Input: dimensioned drawing with shaded views. Units: mm. Origin: part minimum x, y, z. A direction names the side the tool comes from. Coordinates: 2 decimals unless noted, no trailing zeros. Loops run counter-clockwise (first coordinate to the right, second up) from the corner with the lowest first, then second, coordinate; pieces in that order, holes last.
Item 1: Ray query, line 1 along Y through (x, z) = (8, 2.75); line 2 along Y through (x, z) = (4.25, 11.25); line 3 along X through (y, z) = (13.75, 7.5). Return the intervals inside material, ascending.
Item 2: Section B-B on y = 8.5. Return loops of the section in (x, z).
Item 3: Contact query for flat-ended pins moving along their axis: P1, Ø2, axis at x = 4.5, z = 14, coming from the -Y side; P2, Ø1, axis at x = 5.5, z = 8, coming from the +Y side. Output: stop coordinate, or through.
Item 4: Section D-D on x = 3.5. Return loops of the section in (y, z).
Item 5: Section A-A on x = 8.75. Return loops of the section in (y, z).
Item 6: Section C-C on z = 9.75. Give the number of separate pieces and of enclosed holes in the cut face, and give its area (3 significant figures).
Item 7: Reachability of the marked faces 4, 5, 6 and 7 from +Z, -Z, +X, -X, +Y, -Y: full face, straight path, thin tool, end or side. Return the list, or none.
Item 8: Pull-direction query (X, two-part tool) for the marked faces 1, 2 and 3; classes: released by +X, released by -X, zero draft, split by the parting line, or undercut.
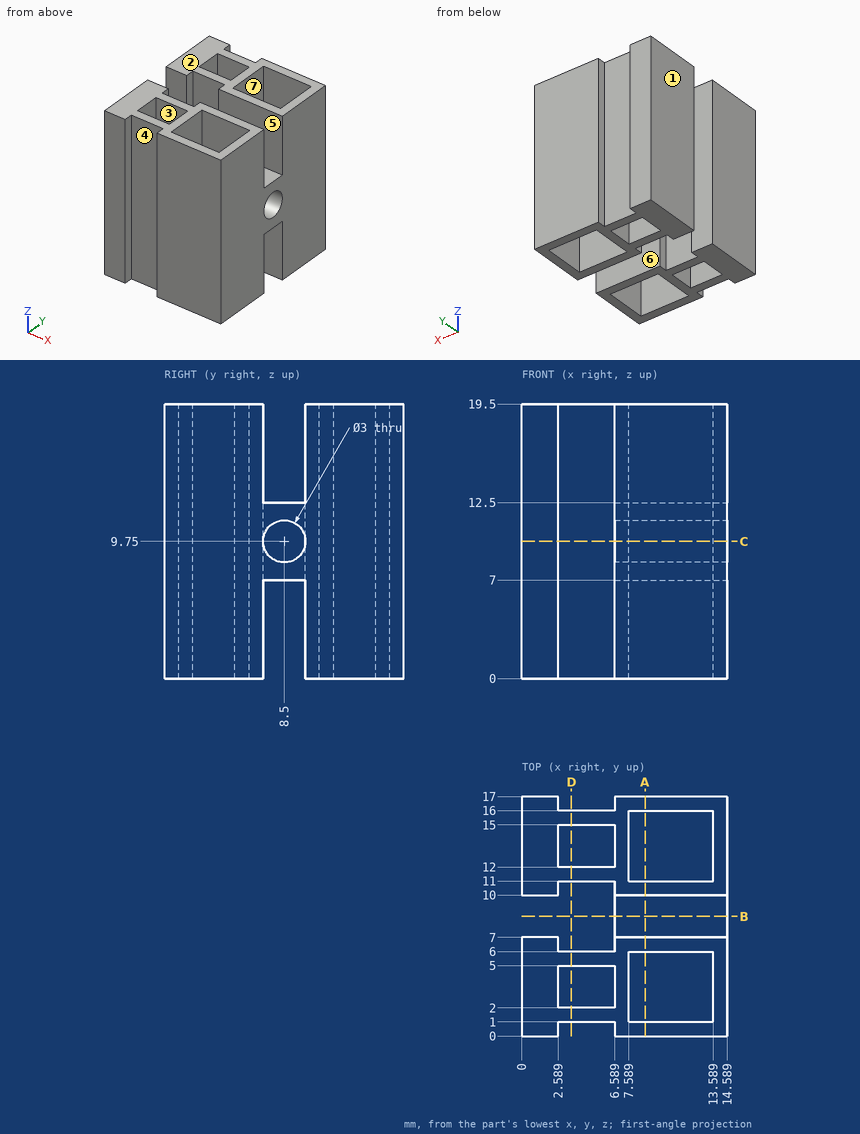
Results found:
1. line 1: y = 0 to 1, 6 to 7, 10 to 11, 16 to 17
1. line 2: y = 1 to 2, 5 to 6, 11 to 12, 15 to 16
1. line 3: x = 0 to 2.59, 6.59 to 7.59, 13.59 to 14.59
2. outline: (6.59, 7) - (14.59, 7) - (14.59, 8.25) - (6.59, 8.25) - close; (6.59, 11.25) - (14.59, 11.25) - (14.59, 12.5) - (6.59, 12.5) - close
3. P1: stops at y = 1
3. P2: stops at y = 16
4. outline: (1, 0) - (2, 0) - (2, 19.5) - (1, 19.5) - close; (5, 0) - (6, 0) - (6, 19.5) - (5, 19.5) - close; (11, 0) - (12, 0) - (12, 19.5) - (11, 19.5) - close; (15, 0) - (16, 0) - (16, 19.5) - (15, 19.5) - close
5. outline: (0, 0) - (1, 0) - (1, 19.5) - (0, 19.5) - close; (6, 0) - (7, 0) - (7, 7) - (10, 7) - (10, 0) - (11, 0) - (11, 19.5) - (10, 19.5) - (10, 12.5) - (7, 12.5) - (7, 19.5) - (6, 19.5) - close; (16, 0) - (17, 0) - (17, 19.5) - (16, 19.5) - close; hole circle Ø3 at (8.5, 9.75)
6. separate pieces: 2
6. enclosed holes: 4
6. area: 104 mm2
7. face 4: +Z, -Z, -Y
7. face 5: +Z, +X, -X
7. face 6: -Z, +X, -X
7. face 7: +Z, -Z
8. face 1: released by -X
8. face 2: zero draft
8. face 3: undercut
